```python
from build123d import *

# Parameters (mm, degrees)
SKETCH052_R             = 1.5
SKETCH052_R_2           = 5
PAD031_DEPTH            = 2
SKETCH053_R             = 14
PAD032_DEPTH            = 30
SKETCH054_R             = 1.5
PAD033_DEPTH            = 14
SKETCH055_R             = 2.5
PAD034_DEPTH            = 26
BODY014_PLACEMENT_ANGLE = 45


with BuildPart() as part:
    # Sketch052 → Pad031 (new body)
    with BuildSketch(Plane.XZ):
        with BuildLine():
            ThreePointArc((3.5, 17.100732), (0, 20.5), (-3.5, 17.100732))
            Line((-3.5, 17.100732), (-3.5, 8.5))
            ThreePointArc((-8.5, 3.5), (-4.964466, 4.964466), (-3.5, 8.5))
            Line((-8.5, 3.5), (-17, 3.5))
            ThreePointArc((-17, 3.5), (-20.5, 0), (-17, -3.5))
            Line((-17, -3.5), (-8.50149, -3.5))
            ThreePointArc((-3.50149, -8.5), (-4.965956, -4.964466), (-8.50149, -3.5))
            Line((-3.50149, -8.5), (-3.50149, -17.002433))
            ThreePointArc((-3.50149, -17.002433), (-0.049155, -20.499656), (3.5, -17.100733))
            Line((3.5, -17.100733), (3.5, -8.5))
            ThreePointArc((8.5, -3.5), (4.964466, -4.964466), (3.5, -8.5))
            Line((8.5, -3.5), (16.999956, -3.5))
            ThreePointArc((16.999956, -3.5), (20.5, -2.2e-05), (17, 3.5))
            Line((17, 3.5), (8.5, 3.5))
            ThreePointArc((3.5, 8.5), (4.964466, 4.964466), (8.5, 3.5))
            Line((3.5, 8.5), (3.5, 17.100732))
        make_face()
        with Locations((0, 16.998507)):
            Circle(SKETCH052_R, mode=Mode.SUBTRACT)
        with Locations((-17, 0)):
            Circle(SKETCH052_R, mode=Mode.SUBTRACT)
        with Locations((17, 0)):
            Circle(SKETCH052_R, mode=Mode.SUBTRACT)
        with Locations((0, -16.420498)):
            Circle(SKETCH052_R, mode=Mode.SUBTRACT)
        Circle(SKETCH052_R_2, mode=Mode.SUBTRACT)
    extrude(amount=PAD031_DEPTH)

    # Sketch053 (on Face23 of Pad031) → Pad032 (join)
    with BuildSketch(Plane.XZ.offset(2)):
        Circle(SKETCH053_R)
    extrude(amount=PAD032_DEPTH)

    # Sketch054 (on Face32 of Pad032) → Pad033 (join)
    with BuildSketch(Plane(origin=(0, -2, 0), x_dir=(1, 0, 0), z_dir=(0, 1, 0))):
        Circle(SKETCH054_R)
    extrude(amount=PAD033_DEPTH)

    # Sketch055 (on Face33 of Pad033) → Pad034 (join)
    with BuildSketch(Plane.XZ.offset(32)):
        Circle(SKETCH055_R)
    extrude(amount=PAD034_DEPTH)


with BuildPart() as part_1:
    # Body014 placement: moved
    add(part.part.moved(Location((-1, -63.5, 22.5))).rotate(Axis((-1, -63.5, 22.5), (0, 1, 0)), BODY014_PLACEMENT_ANGLE))


solid = part_1.part
```
Model file for the job. Use its own axes, mm. A direction names the side the tool comes from. Round coordinates to 2 decimals unless told otherwise and drop trailing zeros. Write each loop counter-clockwise with the first axis right and the second up, starting at its lowest first coordinate (ties: lowest second). Pieces come first, ordered by that corner, then holes. Notation, with made-up numbers: (86.25, 26) - (107.25, 26) arc R27 ccw to (107.25, 57) - close; hole circle Ø6 at (75.5, 64). An arc over 180 degrees is marked (long way). One line per item, written item: value.
(1) Two-plate mould, pull along Z, no slides. Class faces 5 (the cylindrical face through (-15.58, -64.49, 8.09)), 6 (the flat face through (5.5, -64.49, 11.05)), 7 (the cylindrical face through (-14.29, -64.49, 33.72)), 8 (the flat face through (-7.5, -64.49, 33.95)): pulls with the +Z half, pulls with the -Z half, needs draft (parallel to the pull), parting line crosses it, or undercut.
Values follow:
face 5: undercut
face 6: pulls with the -Z half
face 7: undercut
face 8: pulls with the +Z half
(2) 3-axis set-ups, long thin cutter, end or side, ignore diameter. For faces 1 (the flat face through (-11, -65.5, 23)), 2 (the flat face through (-7.62, -64.49, 10.93)), 3 (the flat face through (5.62, -64.49, 34.07)), 4 (the cylindrical face through (6.02, -64.49, 22.55)): which of +Z, -Z, +X, -X, +Y, -Y reach the whole face in a straight line?
Values follow:
face 1: -X, +Y
face 2: -Z, +Y
face 3: +Z, +Y
face 4: +X, +Y
(3) Cut at A-A, the plane x = -1. Give the cut face in (y, z), plus the area to 3 significant figures.
Values follow:
outline: (-121.5, 20) - (-95.5, 20) - (-95.5, 8.5) - (-65.5, 8.5) - (-65.5, 15.48) - (-63.5, 15.48) - (-63.5, 17.5) - (-65.5, 17.5) - (-65.5, 21) - (-51.5, 21) - (-51.5, 24) - (-65.5, 24) - (-65.5, 27.5) - (-63.5, 27.5) - (-63.5, 29.52) - (-65.5, 29.52) - (-65.5, 36.5) - (-95.5, 36.5) - (-95.5, 25) - (-121.5, 25) - close
area: 1,020 mm²
(4) Cut at D-D, the plane y = -96.5. Give the cut face in (x, z).
Values follow:
outline: circle Ø5 at (-1, 22.5)
(5) Cut at C-C, the plane y = -86.5. Give the cut face in (x, z), plus the area to 3 significant figures.
Values follow:
outline: circle Ø28 at (-1, 22.5)
area: 616 mm²
(6) Cut at B-B, the plane z = 22.5. Give the cut face in (x, y).
Values follow:
outline: (-15, -95.5) - (-3.5, -95.5) - (-3.5, -121.5) - (1.5, -121.5) - (1.5, -95.5) - (13, -95.5) - (13, -65.5) - (6.02, -65.5) - (6.02, -63.5) - (4, -63.5) - (4, -65.5) - (0.5, -65.5) - (0.5, -51.5) - (-2.5, -51.5) - (-2.5, -65.5) - (-6, -65.5) - (-6, -63.5) - (-8.02, -63.5) - (-8.02, -65.5) - (-15, -65.5) - close
(7) Wall check: probe 1 along X at (y, z) = (-64.05, 22.5); probe 2 along Z at (x, y) = (-0.5, -72); probe 3 along Y at (x, z) = (-2.5, 29). Give the ranges that are in metal, low to high.
Values follow:
probe 1: x = -8.02 to -6, -2.5 to 0.5, 4 to 6.02
probe 2: z = 8.51 to 36.49
probe 3: y = -95.5 to -63.5
(8) Drop flat-ended pins along their axis: P1, Ø5, axis at x = 4.5, z = 14.5, coming from the -Y side; P2, Ø5, axis at x = 11.02, z = 34.52, coming from the +Y side; P3, Ø4, axis at x = -13.02, z = 34.52, coming from the -Y side; P4, Ø1.8, axis at x = -12.61, z = 10.89, coming from the -Y side. Give the stop position or say it passes through.
Values follow:
P1: stops at y = -95.5
P2: stops at y = -63.5
P3: stops at y = -65.5
P4: passes through
